```python
from build123d import *

# Parameters (mm, degrees)
SKETCH1_W           = 40
SKETCH1_H           = 40.4
BOSS_EXTRUDE1_DEPTH = 20.2
FILLET1_R           = 1
FILLET2_R           = 1
CUT_EXTRUDE1_DEPTH  = 2
SKETCH3_R           = 6.5
BOSS_EXTRUDE2_DEPTH = 0.5
BOSS_EXTRUDE2_TAPER = 20
SKETCH4_R           = 2.25
BOSS_EXTRUDE3_DEPTH = 3.6


with BuildPart() as part:
    # Sketch1 → Boss-Extrude1 (new body)
    with BuildSketch(Plane(origin=(0, 0, 0), x_dir=(1, 0, 0), z_dir=(0, 1, 0))):
        with Locations((20, 20.2)):
            Rectangle(SKETCH1_W, SKETCH1_H)
    extrude(amount=BOSS_EXTRUDE1_DEPTH)

    # Fillet1
    fillet1_edges = [part.edges().sort_by_distance(p)[0] for p in [
        (20, 0, 0),
        (40, 10.1, 0),
        (0, 10.1, 0),
        (20, 20.2, 0),
    ]]
    fillet(fillet1_edges, radius=FILLET1_R)

    # Fillet2
    fillet2_edges = [part.edges().sort_by_distance(p)[0] for p in [
        (20, 20.2, -40.4),
        (20, 0, -40.4),
        (0, 10.1, -40.4),
        (40, 10.1, -40.4),
    ]]
    fillet(fillet2_edges, radius=FILLET2_R)

    # Sketch2 → Cut-Extrude1 (cut)
    with BuildSketch(Plane.XY):
        with BuildLine():
            Line((1.590990258, 3.840990258), (-0.659009742, 3.840990258))
            Line((-0.659009742, 3.840990258), (-0.659009742, 1.590990258))
            ThreePointArc((-0.659009742, 1.590990258), (0, 0), (1.590990258, -0.659009742))
            Line((1.590990258, -0.659009742), (3.840990258, -0.557681221))
            Line((3.840990258, -0.557681221), (3.840990258, 1.590990258))
            ThreePointArc((3.840990258, 1.590990258), (3.181980515, 3.181980515), (1.590990258, 3.840990258))
        make_face()
        with BuildLine():
            Line((3.840990258, 18.609009742), (3.840990258, 20.859009742))
            Line((3.840990258, 20.859009742), (1.590990258, 20.859009742))
            ThreePointArc((1.590990258, 20.859009742), (0, 20.2), (-0.659009742, 18.609009742))
            Line((-0.659009742, 18.609009742), (-0.659009742, 16.359009742))
            Line((-0.659009742, 16.359009742), (1.590990258, 16.359009742))
            ThreePointArc((1.590990258, 16.359009742), (3.181980515, 17.018019485), (3.840990258, 18.609009742))
        make_face()
        with BuildLine():
            Line((36.159009742, -0.557681221), (38.409009742, -0.659009742))
            ThreePointArc((38.409009742, -0.659009742), (40, 0), (40.659009742, 1.590990258))
            Line((40.659009742, 1.590990258), (40.659009742, 3.840990258))
            Line((40.659009742, 3.840990258), (38.409009742, 3.840990258))
            ThreePointArc((38.409009742, 3.840990258), (36.818019485, 3.181980515), (36.159009742, 1.590990258))
            Line((36.159009742, 1.590990258), (36.159009742, -0.557681221))
        make_face()
        with BuildLine():
            Line((36.159009742, 18.609009742), (36.159009742, 20.859009742))
            Line((36.159009742, 20.859009742), (38.409009742, 20.859009742))
            ThreePointArc((38.409009742, 20.859009742), (40, 20.2), (40.659009742, 18.609009742))
            Line((40.659009742, 18.609009742), (40.659009742, 16.359009742))
            Line((40.659009742, 16.359009742), (38.409009742, 16.359009742))
            ThreePointArc((38.409009742, 16.359009742), (36.818019485, 17.018019485), (36.159009742, 18.609009742))
        make_face()
    extrude(amount=-CUT_EXTRUDE1_DEPTH, mode=Mode.SUBTRACT)

    # Sketch3 → Boss-Extrude2 (add)
    with BuildSketch(Plane.XY):
        with Locations((10, 10.1)):
            Circle(SKETCH3_R)
    boss_extrude2 = extrude(amount=BOSS_EXTRUDE2_DEPTH, taper=BOSS_EXTRUDE2_TAPER)

    # Sketch4 → Boss-Extrude3 (add)
    with BuildSketch(Plane.XY.offset(0.5)):
        with Locations((10, 10.1)):
            Circle(SKETCH4_R)
    boss_extrude3 = extrude(amount=BOSS_EXTRUDE3_DEPTH)

    # Mirror2: Boss-Extrude2, Boss-Extrude3 across plane
    add(boss_extrude2.mirror(Plane(origin=(0, 0, -20.2), x_dir=(1, 0, 0), z_dir=(0, 0, -1))))
    add(boss_extrude3.mirror(Plane(origin=(0, 0, -20.2), x_dir=(1, 0, 0), z_dir=(0, 0, -1))))


solid = part.part
```
Input: part model. Units: mm. Frame: model coordinates. A direction names the side the tool comes from. Round coordinates to 2 decimals unless told otherwise and drop trailing zeros. Loops run counter-clockwise (first coordinate to the right, second up) from the corner with the lowest first, then second, coordinate; pieces in that order, holes last. Notation, with made-up numbers: M 39.25,25 L 78.25,25 A4 ccw 78.25,29 Z; hole C 5.5,6.25 d6. An arc over 180 degrees is marked long. Answer in a Markdown table with one row per item. Add a question column.
1. Ray query, probe 1 along Z at (x, y) = (4, 13); probe 2 along Z at (x, y) = (8, 16); probe 3 along X at (y, z) = (17.5, -39.5). Return the intervals inside material, ascending.
2. Section A-A (x = 34). Output: boundary loops of the cut face in (y, z).
3. Section C-C (x = 10). Output: boundary loops of the cut face in (y, z).
4. Section B-B (y = 10.1). Output: boundary loops of the cut face in (x, z).
5. Section D-D (y = 2.5). Output: boundary loops of the cut face in (x, z), and give its area (3 significant figures).
6. Contact query for flat-ended pins moving along their axis: pin 1 (2 mm diameter, centred on y = 4, z = -14.5, fed in from -X); pin 2 (0.5 mm diameter, centred on y = 1, z = -1, fed in from +X); pin 3 (0.8 mm diameter, centred on x = 1, z = -1, fed in from +Y); pin 4 (0.5 mm diameter, centred on x = 1, z = -1, fed in from -Y). Output: stop coordinate, or through.
7. Set-up query: faces 1 (the face through (39, 3.841, -1)), 2 (the face through (3.164, 17.001, -0.986)), 3 (the face through (1, 3.841, -1)), 4 (the face through (39, 16.359, -1)). Return all of +Z, -Z, +X, -X, +Y, -Y with unobstructed straight access to the full face (end or side cutting, diameter ignored); none if empty.
Values follow:
| question | item | result |
|---|---|---|
| 1 | probe 1 | -40.4 to 0 |
| 1 | probe 2 | -40.9 to 0.5 |
| 1 | probe 3 | 0.01 to 39.99 |
| 2 | outline | M 0,-39.4 A1 ccw 1,-40.4 L 19.2,-40.4 A1 ccw 20.2,-39.4 L 20.2,-1 A1 ccw 19.2,0 L 1,0 A1 ccw 0,-1 Z |
| 3 | outline | M 0,-39.4 A1 ccw 1,-40.4 L 3.6,-40.4 L 3.78,-40.9 L 7.85,-40.9 L 7.85,-44.5 L 12.35,-44.5 L 12.35,-40.9 L 16.42,-40.9 L 16.6,-40.4 L 19.2,-40.4 A1 ccw 20.2,-39.4 L 20.2,-1 A1 ccw 19.2,0 L 16.6,0 L 16.42,0.5 L 12.35,0.5 L 12.35,4.1 L 7.85,4.1 L 7.85,0.5 L 3.78,0.5 L 3.6,0 L 1,0 A1 ccw 0,-1 Z |
| 4 | outline | M 0,-39.4 A1 ccw 1,-40.4 L 3.5,-40.4 L 3.68,-40.9 L 7.75,-40.9 L 7.75,-44.5 L 12.25,-44.5 L 12.25,-40.9 L 16.32,-40.9 L 16.5,-40.4 L 39,-40.4 A1 ccw 40,-39.4 L 40,-1 A1 ccw 39,0 L 16.5,0 L 16.32,0.5 L 12.25,0.5 L 12.25,4.1 L 7.75,4.1 L 7.75,0.5 L 3.68,0.5 L 3.5,0 L 1,0 A1 ccw 0,-1 Z |
| 5 | outline | M 0,-39.4 A1 ccw 1,-40.4 L 39,-40.4 A1 ccw 40,-39.4 L 40,-2 L 36.35,-2 L 36.35,0 L 3.65,0 L 3.65,-2 L 0,-2 Z |
| 5 | area | 1,600 mm^2 |
| 6 | pin 1 | x = 0 |
| 6 | pin 2 | x = 36.16 |
| 6 | pin 3 | y = 16.36 |
| 6 | pin 4 | y = 3.84 |
| 7 | face 1 | +Z, +X, -Y |
| 7 | face 2 | +Z, -X, +Y |
| 7 | face 3 | +Z, -X, -Y |
| 7 | face 4 | +Z, +X, +Y |
